from build123d import *

# Parameters (mm, degrees)
BOSS_EXTRUDE1_DEPTH      = 5
BOSS_EXTRUDE2_DEPTH      = 20
FILLET1_R                = 5
F_3_0_3_DIAMETER_HOLE1_D = 3


with BuildPart() as part:
    # Sketch1 → Boss-Extrude1 (new body)
    with BuildSketch(Plane.XY):
        Polygon((-47.026906911, 0), (32.973093089, 1.057571587), (31.842813456, 86.557571587), (-48.157186544, 85.5), align=None)
    extrude(amount=BOSS_EXTRUDE1_DEPTH)

    # Sketch2 → Boss-Extrude2 (add)
    with BuildSketch(Plane.XY):
        Polygon((-33.157186544, 85.698294672), (-33.157186544, 80.698294672), (-13.157186544, 80.698294672), (-13.157186544, 85.962687569), align=None)
        Polygon((11.842813456, 86.29317869), (11.842813456, 81.558008427), (31.908905905, 81.558008427), (31.842813456, 86.557571587), align=None)
        Polygon((-32.092993586, 0.19742103), (-32.092993586, 5.19742103), (-12.092993586, 5.19742103), (-12.092993586, 0.461813927), align=None)
        Polygon((12.907006414, 0.792305048), (12.907006414, 6.056697944), (32.907006414, 6.056697944), (32.907006414, 1.056697944), align=None)
    extrude(amount=BOSS_EXTRUDE2_DEPTH)

    # Fillet1
    fillet1_edges = [part.edges().sort_by_distance(p)[0] for p in [
        (-33.157186544, 83.198294672, 20),
        (-13.157186544, 83.330491121, 20),
        (31.87585968, 84.057790007, 20),
        (11.842813456, 83.925593558, 20),
        (-12.092993586, 2.829617478, 20),
        (-32.092993586, 2.69742103, 20),
        (32.907006414, 3.556697944, 20),
        (12.907006414, 3.424501496, 20),
    ]]
    fillet(fillet1_edges, radius=FILLET1_R)

    # Ø3.0 (3) Diameter Hole1 (through all)
    with Locations(Plane(origin=(-1.138496573, 86.121570382, 0), x_dir=(0.9999126319463549, 0.013218489857519894, 0), z_dir=(-0.013218489857519894, 0.9999126319463549, 0))):
        with Locations((-22.021487627, -15), (22.982444279, -15)):
            Hole(F_3_0_3_DIAMETER_HOLE1_D / 2)


solid = part.part
Check sheet for the modelled part. Datum: model origin and axes. Units: mm. A direction names the side the tool comes from. Round coordinates to 2 decimals unless told otherwise and drop trailing zeros. Loops run counter-clockwise (first coordinate to the right, second up) from the corner with the lowest first, then second, coordinate; pieces in that order, holes last. Notation, with made-up numbers: M -33,15.25 L -5,15.25 A20 ccw -5,51.25 Z; hole C 36.25,12.25 d9. An arc over 180 degrees is marked long. One line per question, with ' | ' between items. Start each with the question number.
Item 1: Scan lines: probe 1 along Y at (x, z) = (17, 19); probe 2 along Y at (x, z) = (27.5, 11.25); probe 3 along Z at (x, y) = (14.5, 72). Record each from-to range of solid material in increasing order.
Item 2: Set-up check for faces 3 (the face through (-23, 80.698, 12)), 4 (the face through (13.27, 83.93, 18.5)): record each of +Z, -Z, +X, -X, +Y, -Y from which the full face is reachable in a straight line by a thin tool's end or side.
Item 3: Section check A-A (z = 8). Record the boundary of the cut face in (x, y), and give its area (3 significant figures).
Item 4: Gauge pin test, flat ends, axial feed: pin 1 Ø24.5 at (x, y) = (4, 37) entering from +Z; pin 2 Ø1.5 at (y, z) = (1.5, 11) entering from -X; pin 3 Ø2.5 at (y, z) = (1.5, 11.5) entering from +X; pin 4 Ø8 at (x, z) = (-5.5, 17.5) entering from -Y. Record the tip position at first contact, or that the pin passes through.
Item 5: Section check C-C (z = 3.75). Record the boundary of the cut face in (x, y), and give its area (3 significant figures).
Item 6: Release check for a two-part mould opening along Y. For faces 1 (the face through (-8, 44, 5)), 2 (the face through (-12.093, 3, 10)) record: released by +Y, released by -Y, zero draft, split by the parting line, or undercut.
Item 7: Section check B-B (x = -29.5). Record the boundary of the cut face in (y, z), and give its area (3 significant figures).
Item 8: Section check D-D (y = 44.5). Record the boundary of the cut face in (x, z), and give its area (3 significant figures).
Worked out:
1) probe 1: 0.85 to 6.06, 81.56 to 86.36 | probe 2: 0.99 to 6.06, 81.56 to 86.5 | probe 3: 0 to 5
2) face 3: +Z, +X, -X | face 4: +Z, +Y, -Y
3) outline: M -33.16,80.7 L -13.16,80.7 L -13.16,85.96 L -33.16,85.7 Z; M -32.09,0.2 L -12.09,0.46 L -12.09,5.2 L -32.09,5.2 Z; M 11.84,81.56 L 31.91,81.56 L 31.84,86.56 L 11.84,86.29 Z; M 12.91,0.79 L 32.91,1.06 L 32.91,6.06 L 12.91,6.06 Z | area: 400 mm^2
4) pin 1: z = 5 | pin 2: x = -32.09 | pin 3: x = 32.91 | pin 4: through
5) outline: M -48.16,85.5 L -47.03,0 L 32.97,1.06 L 31.84,86.56 Z | area: 6,840 mm^2
6) face 1: undercut | face 2: zero draft
7) outline: M 0.23,0 L 85.75,0 L 85.75,19.82 L 80.7,19.82 L 80.7,5 L 5.2,5 L 5.2,19.38 L 0.23,19.38 Z | area: 574 mm^2
8) outline: M -47.62,0 L 32.4,0 L 32.4,5 L -47.62,5 Z | area: 400 mm^2
